```python
from build123d import *

# Parameters (mm, degrees)
F0_R     = 11.1
F1_DEPTH = 7


with BuildPart() as f1:
    # F0 (on Top) → F1 (new body)
    with BuildSketch(Plane.XY):
        with BuildLine():
            Line((10.074664, -12.705239), (31.75576, -12.070901))
            ThreePointArc((31.75576, -12.070901), (32.771356, -11.936183), (33.738175, -11.597295))
            ThreePointArc((33.738175, -11.597295), (33.917325, -11.474048), (34.047629, -11.299963))
            ThreePointArc((34.047629, -11.299963), (36.811106, 0.073562), (33.979335, 11.430276))
            ThreePointArc((33.979335, 11.430276), (33.937596, 11.486441), (33.880845, 11.52738))
            ThreePointArc((33.880845, 11.52738), (32.848475, 11.91711), (31.75576, 12.070901))
            Line((31.75576, 12.070901), (10.074664, 12.705239))
            ThreePointArc((10.074664, 12.705239), (7.72089, 13.372973), (5.965728, 15.077534))
            Line((5.965728, 15.077534), (-5.424174, 33.536745))
            ThreePointArc((-5.424174, 33.536745), (-6.04864, 34.348919), (-6.825536, 35.016764))
            ThreePointArc((-6.825536, 35.016764), (-7.021846, 35.110289), (-7.237759, 35.136093))
            ThreePointArc((-7.237759, 35.136093), (-18.46926, 31.842572), (-26.888577, 23.71183))
            ThreePointArc((-26.888577, 23.71183), (-26.916348, 23.6476), (-26.923426, 23.577983))
            ThreePointArc((-26.923426, 23.577983), (-26.744758, 22.489059), (-26.331587, 21.465845))
            Line((-26.331587, 21.465845), (-16.040392, 2.372295))
            ThreePointArc((-16.040392, 2.372295), (-15.441779, 0), (-16.040392, -2.372295))
            Line((-16.040392, -2.372295), (-26.331587, -21.465845))
            ThreePointArc((-26.331587, -21.465845), (-26.722716, -22.412736), (-26.91264, -23.41947))
            ThreePointArc((-26.91264, -23.41947), (-26.89548, -23.636242), (-26.80987, -23.83613))
            ThreePointArc((-26.80987, -23.83613), (-18.341846, -31.916134), (-7.090758, -35.142106))
            ThreePointArc((-7.090758, -35.142106), (-7.021248, -35.134041), (-6.957419, -35.105362))
            ThreePointArc((-6.957419, -35.105362), (-6.103717, -34.406169), (-5.424174, -33.536745))
            Line((-5.424174, -33.536745), (5.965728, -15.077534))
            ThreePointArc((5.965728, -15.077534), (7.72089, -13.372973), (10.074664, -12.705239))
        make_face()
        with Locations((-11.8, -20.4382)):
            Circle(F0_R, mode=Mode.SUBTRACT)
        Circle(F0_R, mode=Mode.SUBTRACT)
        with Locations((-11.8, 20.4382)):
            Circle(F0_R, mode=Mode.SUBTRACT)
        with Locations((23.6, 0)):
            Circle(F0_R, mode=Mode.SUBTRACT)
    extrude(amount=F1_DEPTH)


solid = f1.part
```
Work out the finished part from the listing and answer in its coordinate system (mm). A direction names the side the tool comes from. Give positions to 0.01 mm unless a question says otherwise; leave off trailing zeros. Loops run counter-clockwise (first coordinate to the right, second up) from the corner with the lowest first, then second, coordinate; pieces in that order, holes last. Notation, with made-up numbers: (19.25, 60) - (49.25, 60) arc R16 cw to (49.25, 64) - close; hole circle Ø4 at (36, -2). An arc over 180 degrees is marked (long way). Use CSV: the item, a comma, the result in double quotes. Start each with the question number.
(1) Find section B-B, the plane x = 4. Determine the outline of the cut face in (y, z), plus the area to 3 significant figures.
(2) Find section D-D, the plane z = 6. Determine the outline of the cut face in (x, y).
(3) Find the intervals of material crossed by L1, parallel to X at y = 2, z = 3.75; L2, parallel to X at y = -0.5, z = 1.25; L3, parallel to X at y = 22, z = 6, in increasing order.
(4) Find section A-A, the plane y = 0. Determine the outline of the cut face in (x, z).
(5) Determine the mould class of faces 1 (the face through (7.69, -13.39, 3.45)), 2 (the face through (32.863, 11.913, 3.451)), 3 (the face through (-6.678, -30.286, 3.451)), 4 (the face through (-26.749, 22.504, 3.451)) for opening direction Y: released by +Y, released by -Y, zero draft, split by the parting line, or undercut.
(6) A tool of negligible diameter and unlimited length cuts with its end or side. For faces 5 (the face through (-26.72, -22.4, 3.45)), 6 (the face through (7.751, 13.356, 3.451)), from which of +Z, -Z, +X, -X, +Y, -Y can it reach the whole face along a straight path? Write none if from no direction.
(7) Each of these flat-tipped pins is pushed along its axis until it touches: pin 1 (13.5 mm diameter, centred on x = 0, y = 0, fed in from -Z); pin 2 (3 mm diameter, centred on y = 18, z = 3, fed in from -X); pin 3 (2 mm diameter, centred on x = -13.5, z = 6, fed in from +Y); pin 4 (2 mm diameter, centred on y = 20.5, z = 3, fed in from -X). Where does it stop, or does it pass through?
(8) Find section C-C, the plane y = 19. Determine the outline of the cut face in (x, z), plus the area to 3 significant figures.
Results found:
1,outline,"(-18.26, 0) - (-10.35, 0) - (-10.35, 7) - (-18.26, 7) - close; (10.35, 0) - (18.26, 0) - (18.26, 7) - (10.35, 7) - close"
1,area,"111 mm^2"
2,outline,"(-26.92, 23.58) arc R5 ccw to (-26.33, 21.47) - (-16.04, 2.37) arc R5 cw to (-16.04, -2.37) - (-26.33, -21.47) arc R5 ccw to (-26.91, -23.42) arc R0.67 ccw to (-26.81, -23.84) arc R24.48 ccw to (-7.09, -35.14) arc R0.23 ccw to (-6.96, -35.11) arc R5 ccw to (-5.42, -33.54) - (5.97, -15.08) arc R5 cw to (10.07, -12.71) - (31.76, -12.07) arc R5 ccw to (33.74, -11.6) arc R0.67 ccw to (34.05, -11.3) arc R24.48 ccw to (33.98, 11.43) arc R0.23 ccw to (33.88, 11.53) arc R5 ccw to (31.76, 12.07) - (10.07, 12.71) arc R5 cw to (5.97, 15.08) - (-5.42, 33.54) arc R5 ccw to (-6.83, 35.02) arc R0.67 ccw to (-7.24, 35.14) arc R24.48 ccw to (-26.89, 23.71) arc R0.23 ccw to start; hole circle Ø22.2 at (-11.8, -20.44); hole circle Ø22.2 at (-11.8, 20.44); hole circle Ø22.2 at (0, 0); hole circle Ø22.2 at (23.6, 0)"
3,L1,"-15.86 to -10.92, 10.92 to 12.68, 34.52 to 36.73"
3,L2,"-15.47 to -11.09, 11.09 to 12.51, 34.69 to 36.81"
3,L3,"-26.58 to -22.79, -0.81 to 1.69"
4,outline,"(-15.44, 0) - (-11.1, 0) - (-11.1, 7) - (-15.44, 7) - close; (11.1, 0) - (12.5, 0) - (12.5, 7) - (11.1, 7) - close; (34.7, 0) - (36.81, 0) - (36.81, 7) - (34.7, 7) - close"
5,face 1,"released by -Y"
5,face 2,"released by +Y"
5,face 3,"undercut"
5,face 4,"undercut"
6,face 5,"+Z, -Z, -X"
6,face 6,"+Z, -Z, +X, +Y"
7,pin 1,"through"
7,pin 2,"x = -25.27"
7,pin 3,"y = 34.33"
7,pin 4,"x = -26.35"
8,outline,"(-25, 0) - (-22.81, 0) - (-22.81, 7) - (-25, 7) - close; (-0.79, 0) - (3.55, 0) - (3.55, 7) - (-0.79, 7) - close"
8,area,"45.7 mm^2"
